The drawing under review shows one solid part. Ordinate dimensions are in mm from its lowest x, y, z. A direction names the side the tool comes from. Coordinates: 2 decimals unless noted, no trailing zeros. Write each loop counter-clockwise with the first axis right and the second up, starting at its lowest first coordinate (ties: lowest second). Pieces come first, ordered by that corner, then holes. Notation, with made-up numbers: M 48,18.25 L 71,18.25 A28 ccw 71,46.25 Z; hole C 56.5,55 d8. An arc over 180 degrees is marked long. Answer as CSV lines item,"result". Start each with the question number.
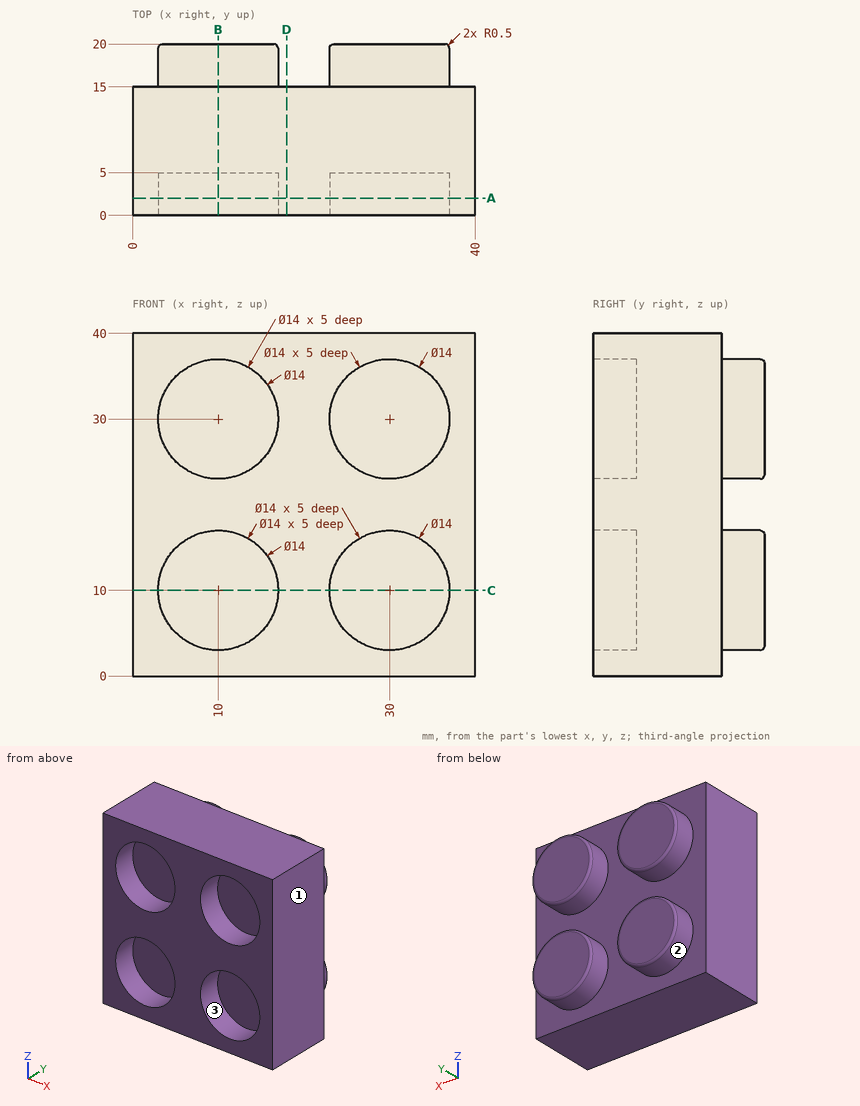
1) Clearance check with flat-ended pins moving along their axes: pin 1 Ø11 at (x, z) = (10, 30) entering from -Y; pin 2 Ø2 at (x, y) = (28, 17) entering from -Z. State where each tip first meets the part, or that it passes through.
2) Take a section at C-C on z = 10. Give the boundary of the cut face in (x, y), and give its area (3 significant figures).
3) Take a section at D-D on x = 18. Give the boundary of the cut face in (y, z).
4) Tool access review of the marked faces 1, 2 and 3: name each direction out of +Z, -Z, +X, -X, +Y, -Y from which nothing blocks a thin tool from reaching the whole face with its end or side.
5) Take a section at A-A on y = 2. Give the boundary of the cut face in (x, z), and give its area (3 significant figures).
6) Take a section at B-B on x = 10. Give the boundary of the cut face in (y, z).
7) To check wall thickness, follow line 1 (Z direction, x = 10, y = 2.35); line 2 (Y direction, x = 20, z = 16); line 3 (Y direction, x = 12, z = 25). State the ranges of each line that lie inside material, in increasing order. Write a range as [from, to].
Results:
1,pin 1,"stops at y = 5"
1,pin 2,"stops at z = 3.07"
2,outline,"M 0,0 L 3,0 L 3,5 L 17,5 L 17,0 L 23,0 L 23,5 L 37,5 L 37,0 L 40,0 L 40,15 L 37,15 L 37,19.5 A0.5 ccw 36.5,20 L 23.5,20 A0.5 ccw 23,19.5 L 23,15 L 17,15 L 17,19.5 A0.5 ccw 16.5,20 L 3.5,20 A0.5 ccw 3,19.5 L 3,15 L 0,15 Z"
2,area,"600 mm²"
3,outline,"M 0,0 L 15,0 L 15,40 L 0,40 Z"
4,face 1,"+Z, -Z, +X, +Y, -Y"
4,face 2,"+Y"
4,face 3,"-Y"
5,outline,"M 0,0 L 40,0 L 40,40 L 0,40 Z; hole C 10,10 d14; hole C 10,30 d14; hole C 30,10 d14; hole C 30,30 d14"
5,area,"984 mm²"
6,outline,"M 0,0 L 15,0 L 15,3 L 19.5,3 A0.5 ccw 20,3.5 L 20,16.5 A0.5 ccw 19.5,17 L 15,17 L 15,23 L 19.5,23 A0.5 ccw 20,23.5 L 20,36.5 A0.5 ccw 19.5,37 L 15,37 L 15,40 L 0,40 L 0,37 L 5,37 L 5,23 L 0,23 L 0,17 L 5,17 L 5,3 L 0,3 Z"
7,line 1,"z = [0, 3], [17, 23], [37, 40]"
7,line 2,"y = [0, 15]"
7,line 3,"y = [5, 20]"
